Part print with two shaded views. Sizes in mm from the minimum x, y, z corner. Coordinates: 2 decimals unless noted, no trailing zeros. Loops run counter-clockwise (first coordinate to the right, second up) from the corner with the lowest first, then second, coordinate; pieces in that order, holes last. Notation, with made-up numbers: (-23, 66.5) - (28, 66.5) arc R12 cw to (28, 89.5) - close; hole circle Ø1 at (65, -1.5). An arc over 180 degrees is marked (long way). Answer as CSV lines item,"result".
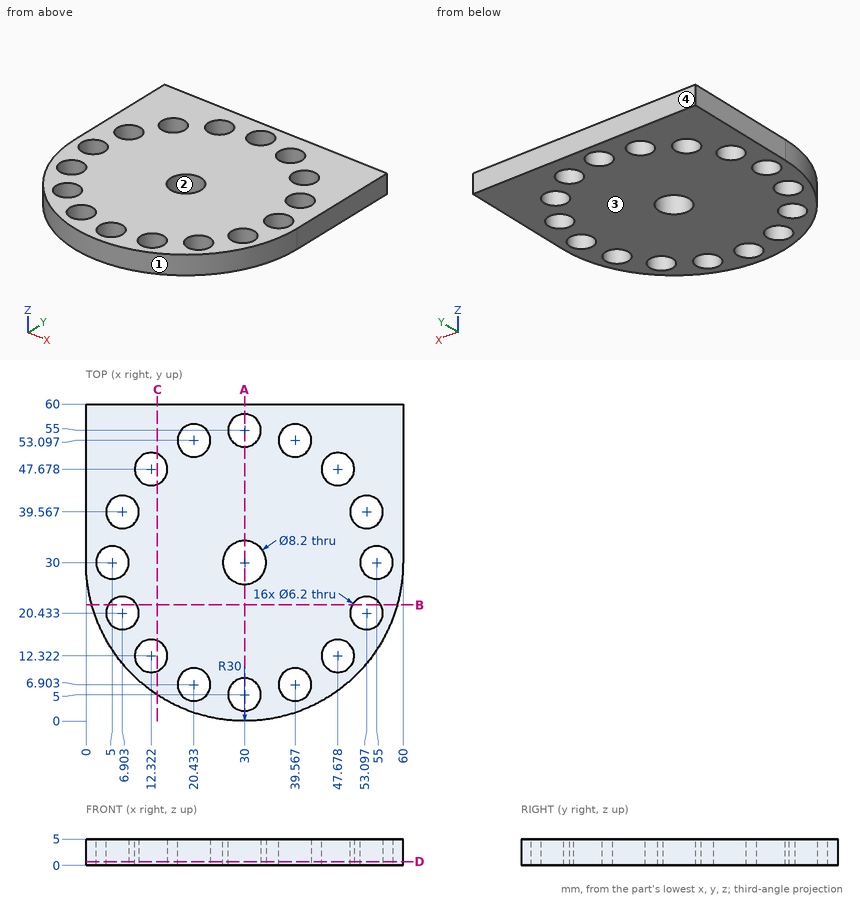
Q1. Flat gauge pin, fed straight in: pin 1 (5 mm diameter, centred on x = 20.43, y = 53.1, fed in from -Z). Where does the tip first touch, or does it go through?
Results:
pin 1,"passes through"
Q2. Two-plate mould, pull along Y, no slides. Class the marked faces 1, 2, 3 and 4: released by +Y, released by -Y, zero draft, split by the parting line, or undercut.
Results:
face 1,"released by -Y"
face 2,"undercut"
face 3,"zero draft"
face 4,"released by +Y"
Q3. Saw through at A-A (x = 30). Give the cut face in (y, z), then the cut area to 3 significant figures.
Results:
outline,"(0, 0) - (1.9, 0) - (1.9, 5) - (0, 5) - close; (8.1, 0) - (25.9, 0) - (25.9, 5) - (8.1, 5) - close; (34.1, 0) - (51.9, 0) - (51.9, 5) - (34.1, 5) - close; (58.1, 0) - (60, 0) - (60, 5) - (58.1, 5) - close"
area,"197 mm^2"
Q4. Wall check: L1, parallel to Y at x = 30, z = 3.7; L2, parallel to Y at x = 47, z = 2.3; L3, parallel to Y at x = 49, z = 0.7 (1 decimal). Give the ranges that are in metal, low to high.
Results:
L1,"y = 0 to 1.9, 8.1 to 25.9, 34.1 to 51.9, 58.1 to 60"
L2,"y = 5.28 to 9.3, 15.35 to 44.65, 50.7 to 60"
L3,"y = 6.8 to 9.5, 15.1 to 44.9, 50.5 to 60"
Q5. Saw through at D-D (z = 0.7). Count the separate pieces of the cut face and the enclosed holes in it, then the cut area to 3 significant figures.
Results:
separate pieces,"1"
enclosed holes,"17"
area,"2,680 mm^2"
Q6. Saw through at B-B (y = 22). Give the cut face in (x, z).
Results:
outline,"(1.09, 0) - (4.23, 0) - (4.23, 5) - (1.09, 5) - close; (9.58, 0) - (50.42, 0) - (50.42, 5) - (9.58, 5) - close; (55.77, 0) - (58.91, 0) - (58.91, 5) - (55.77, 5) - close"
Q7. Saw through at C-C (x = 13.5). Give the cut face in (y, z) (1 decimal), then the cut area to 3 significant figures.
Results:
outline,"(4.9, 0) - (9.5, 0) - (9.5, 5) - (4.9, 5) - close; (15.2, 0) - (44.8, 0) - (44.8, 5) - (15.2, 5) - close; (50.5, 0) - (60, 0) - (60, 5) - (50.5, 5) - close"
area,"218 mm^2"
